```python
from build123d import *

# Parameters (mm, degrees)
BOSS_EXTRUDE1_DEPTH = 20
SKETCH2_R           = 2.5
CUT_EXTRUDE1_DEPTH  = 20
SKETCH3_R           = 2.5
CUT_EXTRUDE2_DEPTH  = 20
SKETCH4_R           = 2.5
CUT_EXTRUDE3_DEPTH  = 20
SKETCH5_R           = 4
CUT_EXTRUDE4_DEPTH  = 5


with BuildPart() as part:
    # Sketch1 → Boss-Extrude1 (new body)
    with BuildSketch(Plane.XY):
        with BuildLine():
            Line((85, 232.5), (135, 232.5))
            Line((135, 232.5), (135, -232.5))
            Line((135, -232.5), (85, -232.5))
            Line((85, -232.5), (85, -152.5))
            ThreePointArc((85, -152.5), (70.355339059, -117.144660941), (35, -102.5))
            Line((35, -102.5), (-35, -102.5))
            ThreePointArc((-35, -102.5), (-70.355339059, -117.144660941), (-85, -152.5))
            Line((-85, -152.5), (-85, -232.5))
            Line((-85, -232.5), (-135, -232.5))
            Line((-135, -232.5), (-135, 232.5))
            Line((-135, 232.5), (-85, 232.5))
            Line((-85, 232.5), (-85, 150))
            ThreePointArc((-85, 150), (-70.355339059, 114.644660941), (-35, 100))
            Line((-35, 100), (35, 100))
            ThreePointArc((35, 100), (70.355339059, 114.644660941), (85, 150))
            Line((85, 150), (85, 232.5))
        make_face()
    extrude(amount=BOSS_EXTRUDE1_DEPTH)

    # Sketch2 → Cut-Extrude1 (cut)
    with BuildSketch(Plane.XZ.offset(232.5)):
        with Locations((-120, 10)):
            Circle(SKETCH2_R)
        with Locations((-100, 10)):
            Circle(SKETCH2_R)
        with Locations(Location((100, 10, 0), (0, 0, 180))):
            Circle(SKETCH2_R)
        with Locations(Location((120, 10, 0), (0, 0, 180))):
            Circle(SKETCH2_R)
    cut_extrude1 = extrude(amount=-CUT_EXTRUDE1_DEPTH, mode=Mode.SUBTRACT)

    # Mirror1: Cut-Extrude1 across plane
    add(cut_extrude1.mirror(Plane.ZX), mode=Mode.SUBTRACT)

    # Sketch3 → Cut-Extrude2 (cut)
    with BuildSketch(Plane.XY.offset(20)):
        with Locations((100, 85)):
            Circle(SKETCH3_R)
        with Locations(Location((100, -85, 0), (0, 0, 180))):
            Circle(SKETCH3_R)
        with Locations(Location((-100, 85, 0), (0, 0, 180))):
            Circle(SKETCH3_R)
        with Locations((-100, -85)):
            Circle(SKETCH3_R)
    extrude(amount=-CUT_EXTRUDE2_DEPTH, mode=Mode.SUBTRACT)

    # Sketch4 → Cut-Extrude3 (cut)
    with BuildSketch(Plane(origin=(0, 0, 0), x_dir=(-1, 0, 0), z_dir=(0, 0, -1))):
        with Locations((-110, 4.5)):
            Circle(SKETCH4_R)
        with Locations(Location((-110, -4.5, 0), (0, 0, 180))):
            Circle(SKETCH4_R)
        with Locations((15, 4.5)):
            Circle(SKETCH4_R)
        with Locations(Location((15, -4.5, 0), (0, 0, 180))):
            Circle(SKETCH4_R)
    extrude(amount=-CUT_EXTRUDE3_DEPTH, mode=Mode.SUBTRACT)

    # Sketch5 → Cut-Extrude4 (cut)
    with BuildSketch(Plane(origin=(0, 0, 0), x_dir=(-1, 0, 0), z_dir=(0, 0, -1))):
        with Locations((-110, 4.5)):
            Circle(SKETCH5_R)
        with Locations((-110, -4.5)):
            Circle(SKETCH5_R)
        with Locations(Location((15, 4.5, 0), (0, 0, 180))):
            Circle(SKETCH5_R)
        with Locations(Location((15, -4.5, 0), (0, 0, 180))):
            Circle(SKETCH5_R)
    extrude(amount=-CUT_EXTRUDE4_DEPTH, mode=Mode.SUBTRACT)


solid = part.part
```
Check sheet for the modelled part. Datum: model origin and axes. Units: mm. A direction names the side the tool comes from. Round coordinates to 2 decimals unless told otherwise and drop trailing zeros. Order: outer loops, then holes, each group sorted by start corner. A loop starts at its lowest first (then second) coordinate and runs counter-clockwise, first axis right, second up.
1) Scan lines: line 1 (X direction, y = -4.5, z = 17); line 2 (Y direction, x = -15, z = 8.75); line 3 (Y direction, x = -100, z = 13.5). Record each from-to range of solid material in increasing order.
2) Tool access check on faces 1 (the cylindrical face through (-69.964, -116.758, 9.86)), 2 (the cylindrical face through (69.964, 114.258, 9.86)), 3 (the flat face through (-110, -232.5, 10)). Record the directions out of +Z, -Z, +X, -X, +Y, -Y that give a thin tool (end or side, any length) a straight path to the whole face; none if there is none.
3) Section check B-B (x = -41.5). Record the boundary of the cut face in (y, z), and give its area (3 significant figures).
4) Section check A-A (y = -147). Record the boundary of the cut face in (x, z).
5) Section check C-C (x = -77.5). Record the boundary of the cut face in (y, z).
6) Go/stop test with flat-tipped pins: pin 1 Ø4.5 at (x, z) = (-100, 10) entering from -Y; pin 2 Ø8 at (x, z) = (-59, 11) entering from +Y; pin 3 Ø5 at (x, z) = (-9.5, 18) entering from -Y; pin 4 Ø4.5 at (x, y) = (110, -4.5) entering from +Z. Record where each tip stops, or that it passes through.
7) Mould release check, pull along X, two halves, no side actions. Record for faces 4 (the cylindrical face through (70.742, -117.536, 9.86)), 5 (the flat face through (135, 3, 10)), 6 (the flat face through (2, 3, 20)): +X half, -X half, draft (parallel to the pull), parting line (faces both ways), or undercut.
Result:
1. line 1: x = -135 to -17.5, -12.5 to 107.5, 112.5 to 135
1. line 2: y = -102.5 to -7, -2 to 2, 7 to 100
1. line 3: y = -232.5 to -87.5, -82.5 to 82.5, 87.5 to 232.5
2. face 1: +Z, -Z, -Y
2. face 2: +Z, -Z, +Y
2. face 3: +Z, -Z, +X, -X, -Y
3. outline: (-102.92, 0) - (100.42, 0) - (100.42, 20) - (-102.92, 20) - close
3. area: 4,070 mm2
4. outline: (-135, 0) - (-84.7, 0) - (-84.7, 20) - (-135, 20) - close; (84.7, 0) - (135, 0) - (135, 20) - (84.7, 20) - close
5. outline: (-126.16, 0) - (123.66, 0) - (123.66, 20) - (-126.16, 20) - close
6. pin 1: stops at y = -212.5
6. pin 2: stops at y = 108.58
6. pin 3: stops at y = -102.5
6. pin 4: passes through
7. face 4: undercut
7. face 5: +X half
7. face 6: draft
